The model under review builds one solid part; all positions refer to its coordinate system, in mm. A direction names the side the tool comes from. Give positions to 0.01 mm unless a question says otherwise; leave off trailing zeros. Loops run counter-clockwise (first coordinate to the right, second up) from the corner with the lowest first, then second, coordinate; pieces in that order, holes last. Notation, with made-up numbers: M -16.5,-22.5 L 9.5,-22.5 A11 cw 9.5,-3.5 Z; hole C 71.25,-11.75 d2. An arc over 180 degrees is marked long. Put each result on its own line as item: value. Start each with the question number.
Autodesk Inventor part; units mm, degrees
ref_plane "YZ Plane" through (0, 0, 0) normal (1, 0, 0) x (0, 1, 0)
ref_plane "XZ Plane" through (0, 0, 0) normal (0, 1, 0) x (-1, 0, 0)
ref_plane "XY Plane" through (0, 0, 0) normal (0, 0, 1) x (1, 0, 0)
sketch "Sketch1" plane through (0, 0, 0) normal (0, 0, 1) x (1, 0, 0)
  line L0 (254.7886, 18.124) -> (254.7886, 0) construction
  line L1 (192, 54.375) -> (254.7886, 18.124)
  line L2 (0, 0) -> (487.78, 0)
  line L3 (254.7886, 18.124) -> (256.7886, 18.124)
  line L4 (256.7886, 18.124) -> (327.1228, 36.97)
  line L5 (327.1228, 36.97) -> (327.1228, 0)
  line L6 (327.1228, 40.0758) -> (255.8936, 20.258)
  line L7 (255.8936, 20.258) -> (255.0924, 20.258)
  line L8 (255.0924, 20.258) -> (192.3194, 56.5)
  line L9 (327.1228, 36.97) -> (327.1228, 40.0758)
  line L10 (192, 54.375) -> (191.7835, 54.5)
  line L11 (0, 0) -> (0, 54.5)
  line L12 (0, 54.5) -> (274.8621, 54.5) construction
  line L13 (191.7835, 54.5) -> (188.7835, 54.5)
  line L14 (188.7835, 54.5) -> (188.7835, 56.5)
  line L15 (188.7835, 56.5) -> (192.3194, 56.5)
  line L16 (327.1228, 0) -> (327.1228, 59.5)
  line L17 (327.1228, 59.5) -> (323.1228, 59.5)
  line L18 (323.1228, 59.5) -> (319.1228, 59.5)
  line L19 (319.1228, 59.5) -> (319.1228, 37.85)
  line L20 (188.7835, 54.5) -> (188.7835, 0)
  point P0 (322.4487, 38.7754)
  point P1 (191.9595, 55.4142)
  point P2 (188.9595, 55.4)
  point P3 (323.1228, 38.9629)
  dimension "d2" = 18.124
  dimension "d4" = 30
  dimension "d5" = 18.124
  dimension "d6" = 2
  dimension "d7" = 15
  dimension "d8" = 36.97
  dimension "d9" = 2
  dimension "d19" = 54.5
  dimension "d20" = 3
  dimension "d21" = 2
  dimension "d22" = 59.5
  dimension "d23" = 4
  dimension "d24" = 4
revolve "Revolution1" add sketch "Sketch1" angle 360 about axis through (0, 0, 0) along (1, 0, 0) contours L10 L13 L14 L15 L8 L7 L6 L9 L4 L3 L1 | L6 L19 L18 L17 L16
sketch "Sketch2" plane through (0, 0, 0) normal (0, 0, 1) x (1, 0, 0)
  line L0 (319.1228, -59.5) -> (319.1228, 59.5)
  line L1 (319.1228, 59.5) -> (322.1228, 59.5)
  line L2 (319.1228, 59.5) -> (327.1228, 59.5)
  line L3 (322.1228, 59.5) -> (324.1228, 59.5)
  line L4 (324.1228, 59.5) -> (324.1228, 57.5)
  line L5 (324.1228, 57.5) -> (322.1228, 57.5)
  line L6 (322.1228, 57.5) -> (322.1228, 59.5)
  line L7 (-65.4246, 0) -> (392.5474, 0)
  point P0 (0, 0)
  dimension "d25" = 3
  dimension "d26" = 2
  dimension "d27" = 2
revolve "Revolution2" cut sketch "Sketch2" angle 360 about axis through (-10, 0, 0) along (1, 0, 0)
properties part number "stainless steel final nozzle" material "Stainless Steel"
Item 1: Clearance check with flat-ended pins moving along their axes: pin 1 Ø6 at (x, z) = (285, 27) entering from +Y; pin 2 Ø2 at (x, y) = (279, 7) entering from -Z; pin 3 Ø8 at (x, z) = (236.5, 12.5) entering from -Y. State where each tip first meets the part, or that it passes through.
Item 2: Draft analysis for pull direction X (two halves, no side actions). For faces 1 (the cylindrical face through (255.487, -4.392, 19.776)), 2 (the cylindrical face through (323.109, -12.465, 56.133)), 3 (the flat face through (188.784, -30, 46)), 4 (the flat face through (327.123, -27, -26)), state which applies: +X half, -X half, draft (parallel to the pull), parting line (faces both ways), or undercut.
Item 3: Consider section C-C, the plane x = 244. Write out the cut boundary in (y, z), plus the area to 3 significant figures.
Item 4: Consider section D-D, the plane x = 271. Write out the cut boundary in (y, z), plus the area to 3 significant figures.
Item 5: Tool access review of faces 5 (the cylindrical face through (255.8, -14.38, -11.03)), 6 (the flat face through (319.123, -1, -39)), 7 (the cylindrical face through (190.26, -43.25, 33.16)): name each direction out of +Z, -Z, +X, -X, +Y, -Y from which nothing blocks a thin tool from reaching the whole face with its end or side.
Item 6: To check wall thickness, follow L1, parallel to X at y = 24.5, z = -53; L2, parallel to Z at x = 190, y = 0; L3, parallel to Z at x = 255.35, y = 0. State the ranges of each line that lie inside material, in increasing order. Write a range as [from, to].
Report:
1. pin 1: y = 15.35
1. pin 2: z = -26.14
1. pin 3: y = -31.28
2. face 1: undercut
2. face 2: undercut
2. face 3: -X half
2. face 4: +X half
3. outline: C 0,0 d53.32; hole C 0,0 d48.71
3. area: 370 mm²
4. outline: C 0,0 d48.92; hole C 0,0 d43.86
4. area: 369 mm²
5. face 5: +X, -X
5. face 6: none
5. face 7: -X
6. L1: [319.12, 322.12], [324.12, 327.12]
6. L2: [-56.5, -54.5], [54.5, 56.5]
6. L3: [-20.26, -18.12], [18.12, 20.26]
